Read the model definition and answer for the solid it produces. Units are mm, in the model's axes. A direction names the side the tool comes from. Coordinates: 2 decimals unless noted, no trailing zeros. Write each loop counter-clockwise with the first axis right and the second up, starting at its lowest first coordinate (ties: lowest second). Pieces come first, ordered by that corner, then holes.
1) Find the intervals of material crossed by line 1 (Y direction, x = -1.15, z = 0.5); line 2 (Z direction, x = 1.25, y = 1); line 3 (Z direction, x = -0.8, y = 4), in increasing order.
2) The part is cut by section A-A (y = 6.5). Determine the outline of the cut face in (x, z).
3) Each of these flat-tipped pins is pushed along its axis until it touches: pin 1 Ø1.5 at (y, z) = (4, -0.5) entering from -X; pin 2 Ø1.5 at (x, y) = (0, 6.5) entering from +Z; pin 3 Ø1.2 at (x, z) = (-0.5, 0.5) entering from +Y. Where does it stop, or does it pass through?
4) Which of the six approach directions +Z, -Z, +X, -X, +Y, -Y give full straight-line access (tool end or side, diameter ignored) to faces 1 (the face through (-1, 4, 0)), 2 (the face through (0, 0, 0))?
from build123d import *

# Parameters (mm, degrees)
SKETCH_1_R      = 1.725
EXTRUDE_1_DEPTH = 1.17
FILLET_1_R      = 0.5
SKETCH_2_R      = 1
EXTRUDE_2_DEPTH = 8
CHAMFER_1_SIZE  = 1.7
CHAMFER_1_SIZE2 = 0.981495458


with BuildPart() as part:
    # 草图1 → 凸台-拉伸1 (new body)
    with BuildSketch(Plane(origin=(0, 0, 0), x_dir=(1, 0, 0), z_dir=(0, 1, 0))):
        with Locations(Location((0, 0, 0), (0, 0, 90))):
            Circle(SKETCH_1_R)
    extrude(amount=EXTRUDE_1_DEPTH)

    # 圆角1
    fillet_1_edges = [part.edges().sort_by_distance(p)[0] for p in [
        (0, 0, 1.725),
        (0, 1.17, 1.725),
    ]]
    fillet(fillet_1_edges, radius=FILLET_1_R)

    # 草图2 → 凸台-拉伸2 (add)
    with BuildSketch(Plane(origin=(0, 1.17, 0), x_dir=(1, 0, 0), z_dir=(0, 1, 0))):
        with Locations(Location((0, 0, 0), (0, 0, 270))):
            Circle(SKETCH_2_R)
    extrude(amount=EXTRUDE_2_DEPTH)

    # 倒角1
    chamfer_1_edges = [part.edges().sort_by_distance(p)[0] for p in [
        (0, 9.17, -1),
    ]]
    chamfer_1_side = [part.faces().sort_by_distance(p)[0] for p in [
        (0, 5.17, -1),
    ]]
    chamfer(chamfer_1_edges, length=CHAMFER_1_SIZE, length2=CHAMFER_1_SIZE2, reference=chamfer_1_side[0])


solid = part.part
Reported:
1. line 1: y = 0 to 1.17
1. line 2: z = -1 to 1
1. line 3: z = -0.6 to 0.6
2. outline: circle Ø2 at (0, 0)
3. pin 1: stops at x = -1
3. pin 2: stops at z = 1
3. pin 3: stops at y = 9.02
4. face 1: +Y
4. face 2: +Z, -Z, +X, -X, -Y
